Can you work these out from the model? Positions are in its coordinate system, mm. Coordinates: 2 decimals unless noted, no trailing zeros. Order: outer loops, then holes, each group sorted by start corner. A loop starts at its lowest first (then second) coordinate and runs counter-clockwise, first axis right, second up. Notation, with made-up numbers: (44.5, -35) - (88.5, -35) arc R23 cw to (88.5, -9) - close; hole circle Ø5 at (5.25, -18). An arc over 180 degrees is marked (long way). Return JSON: item names as keys, results as strings. Group by question number.
1) Imagine slicing it at C-C (z = 383). Write out the boundary of the cut face in (x, y).
2) For pin 1 Ø8 at (x, y) = (-12.5, 15.5) entering from -Z, with a flat end and sliding along its axis, tell me the tip position at first contact or that it passes through.
3) Imagine slicing it at A-A (y = 15). Write out the boundary of the cut face in (x, z).
4) Imagine slicing it at B-B (x = -5). Write out the boundary of the cut face in (y, z).
5) If I drill on line 1 along Y through (x, z) = (-10.5, 558); line 2 along X through (y, z) = (-22.5, 524); line 3 along Y through (x, z) = (-15, 112.5), over which ranges is the centre line in solid material (lowest first)?
Autodesk Inventor part; units mm, degrees
ref_plane "Start plane" through (0, 0, 0) normal (0, 0, 1) x (1, 0, 0)
ref_plane "End plane" through (0, 0, 1000) normal (0, 0, 1) x (1, 0, 0)
ref_plane "YZ Plane" through (0, 0, 0) normal (1, 0, 0) x (0, 1, 0)
ref_plane "Start plane" through (0, 0, 0) normal (0, 0, 1) x (1, 0, 0)
ref_plane "End plane" through (0, 0, 1000) normal (0, 0, 1) x (1, 0, 0)
sketch "Sketch" plane through (0, 0, 0) normal (0, 0, 1) x (1, 0, 0)
  line L0 (-20, -24) -> (-20, 24)
  line L1 (-14, 30) -> (14, 30)
  line L2 (20, 24) -> (20, -24)
  line L3 (14, -30) -> (-14, -30)
  arc A0 (-20, -24) -> (-14, -30) centre (-14, -24) ccw
  arc A1 (20, 24) -> (14, 30) centre (14, 24) ccw
  arc A2 (-14, 30) -> (-20, 24) centre (-14, 24) ccw
  arc A3 (14, -30) -> (20, -24) centre (14, -24) ccw
  arc A4 (-14, 27) -> (-17, 24) centre (-14, 24) ccw
  line L4 (-14, 27) -> (14, 27)
  arc A5 (17, 24) -> (14, 27) centre (14, 24) ccw
  line L5 (17, 24) -> (17, -24)
  arc A6 (14, -27) -> (17, -24) centre (14, -24) ccw
  line L6 (14, -27) -> (-14, -27)
  arc A7 (-17, -24) -> (-14, -27) centre (-14, -24) ccw
  line L7 (-17, -24) -> (-17, 24)
  line L8 (0, 37.1021) -> (0, -37.1021) construction
  line L9 (-23.1021, 0) -> (23.1021, 0) construction
  dimension "d7" = 6
  dimension "d9" = 40
  dimension "d11" = 60
  dimension "d12" = 3
  dimension "d15" = 20
  dimension "d16" = 30
extrude "Body" add sketch "Sketch" along normal up to surface (1000 mm away) from surface at 0
sketch "Sketch3" plane through (0, 0, 0) normal (0, 0, 1) x (1, 0, 0)
  line L0 (0, 0) -> (10, 0)
ref_plane "Work Plane3" through (0, 0, 0) normal (0, -1, 0) x (1, 0, 0)
sketch "Sketch5" plane through (20, -24, 1000) normal (1, 0, 0) x (0, 0, -1)
  line L0 (0, 0) -> (0, -6)
  line L1 (1000, -6) -> (0, -6)
  line L2 (1000, 0) -> (1000, -6)
  line L3 (1000, 0) -> (0, 0)
  line L4 (0, 48) -> (0, 0)
  line L5 (1000, 0) -> (0, 0)
  line L6 (1000, 48) -> (1000, 0)
  line L7 (1000, 48) -> (0, 48)
  line L8 (0, 54) -> (0, 48)
  line L9 (1000, 48) -> (0, 48)
  line L10 (1000, 54) -> (1000, 48)
  line L11 (1000, 54) -> (0, 54)
  line L12 (0, 54) -> (60, -6)
  line L13 (1000, 54) -> (940, -6)
  line L14 (1000, -6) -> (0, -6)
  point P0 (1000, 24)
  dimension "d19" = 45
  dimension "d20" = 45
extrude "Extrusion2" cut sketch "Sketch5" against normal through all contours L3 L12 L1 L0 | L4 L7 L12 L3 | L8 L12 L7 | L13 L7 L6 L3 | L3 L2 L1 L13 | L13 L10 L7
sketch "Sketch4" plane through (0, 0, 0) normal (0, -1, 0) x (1, 0, 0)
  line L0 (-2, 0) -> (12, 0)
  line L1 (-2, 1000) -> (12, 1000)
  dimension "d18" = 1000
equation "\"d7\" = G_IR"
equation "\"d9\" = G_W"
equation "\"d11\" = G_H"
equation "\"d12\" = G_T"
equation "\"d15\" = 0.5 * d9"
equation "\"d16\" = 0.5 * d11"
equation "\"d3\" = G_L"
equation "\"d20\" = d19"
equation "\"G_W\" = 40"
equation "\"G_H\" = 60"
equation "\"G_T\" = 3"
equation "\"G_IR\" = 6"
equation "\"G_L\" = d18"
equation "\"G_OFFSET_START\" = 0"
equation "\"G_OFFSET_END\" = 0"
properties part number "ISO 4019 - 60x40x3 - 1000" material "Steel, Mild"
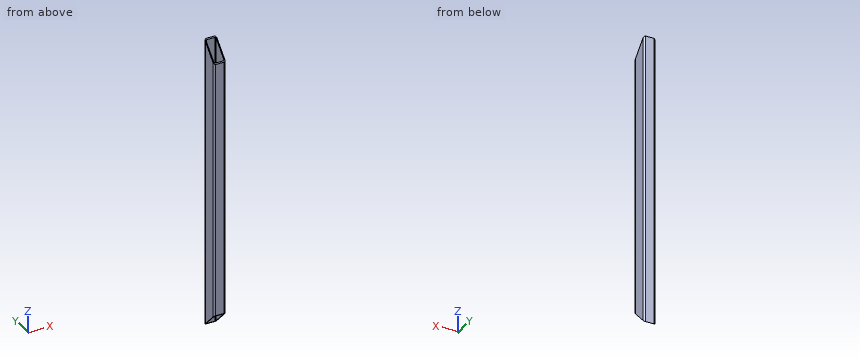
Calculated:
{
 "1": {"outline": "(-20, -24) arc R6 ccw to (-14, -30) - (14, -30) arc R6 ccw to (20, -24) - (20, 24) arc R6 ccw to (14, 30) - (-14, 30) arc R6 ccw to (-20, 24) - close; hole (-17, -24) arc R3 ccw to (-14, -27) - (14, -27) arc R3 ccw to (17, -24) - (17, 24) arc R3 ccw to (14, 27) - (-14, 27) arc R3 ccw to (-17, 24) - close"},
 "2": {"pin 1": "through"},
 "3": {"outline": "(-20, 15) - (-17, 15) - (-17, 985) - (-20, 985) - close; (17, 15) - (20, 15) - (20, 985) - (17, 985) - close"},
 "4": {"outline": "(-30, 60) - (-27, 57) - (-27, 943) - (-30, 940) - close; (27, 3) - (30, 0) - (30, 1000) - (27, 997) - close"},
 "5": {"line 1": "-30 to -27, 27 to 30", "line 2": "-20 to -17, 17 to 20", "line 3": "-29.92 to -26.83, 26.83 to 29.92"}
}
